Autodesk Inventor part; units mm, degrees
ref_plane "YZ Plane" through (0, 0, 0) normal (1, 0, 0) x (0, 1, 0)
ref_plane "XZ Plane" through (0, 0, 0) normal (0, 1, 0) x (-1, 0, 0)
ref_plane "XY Plane" through (0, 0, 0) normal (0, 0, 1) x (1, 0, 0)
sketch "Sketch1" plane through (0, 0, 0) normal (0, 1, 0) x (-1, 0, 0)
  circle A0 centre (0, 0) radius 76.2
  circle A1 centre (0, 0) radius 82.55
  line L0 (0, 0) -> (101.6, 0)
  arc A2 (82.55, 0) -> (101.6, 0) centre (92.075, 26.1697) ccw
  line L1 (101.6, 0) -> (92.4836, -3.3181) construction
  arc A3 (93.6625, -13.7482) -> (101.6, 0) centre (85.725, 0) ccw
  line L2 (93.6625, -13.7482) -> (79.6013, -21.8664)
  arc A4 (92.075, -10.9985) -> (98.3891, -0.9543) centre (85.725, 0) ccw
  line L3 (92.075, -10.9985) -> (80.6536, -17.5927)
  arc A5 (82.4826, -3.3343) -> (101.2144, -3.4778) centre (92.075, 26.1697) ccw
  arc A6 (-41.275, 71.4904) -> (-50.8, 87.9882) centre (-68.7011, 66.6544) ccw
  line L4 (-50.8, 87.9882) -> (-43.3683, 81.7522) construction
  arc A7 (-34.925, 87.9882) -> (-50.8, 87.9882) centre (-42.8625, 74.24) ccw
  line L5 (-34.925, 87.9882) -> (-20.8638, 79.8699)
  arc A8 (-36.5125, 85.2386) -> (-48.3681, 85.6846) centre (-42.8625, 74.24) ccw
  line L6 (-36.5125, 85.2386) -> (-25.0911, 78.6444)
  arc A9 (-38.3537, 73.0992) -> (-47.5953, 89.3931) centre (-68.7011, 66.6544) ccw
  arc A10 (-41.275, -71.4904) -> (-50.8, -87.9882) centre (-23.3739, -92.8242) ccw
  line L7 (-50.8, -87.9882) -> (-49.1154, -78.4341) construction
  arc A11 (-58.7375, -74.24) -> (-50.8, -87.9882) centre (-42.8625, -74.24) ccw
  line L8 (-58.7375, -74.24) -> (-58.7375, -58.0035)
  arc A12 (-55.5625, -74.24) -> (-50.021, -84.7303) centre (-42.8625, -74.24) ccw
  line L9 (-55.5625, -74.24) -> (-55.5625, -61.0517)
  arc A13 (-44.1289, -69.7649) -> (-53.619, -85.9153) centre (-23.3739, -92.8242) ccw
  point P0 (-20.8638, 79.8699)
  point P1 (-41.275, 71.4904)
  point P2 (-58.7375, -58.0035)
  point P3 (-41.275, -71.4904)
  point P4 (-44.1289, -69.7649)
  point P5 (-52.5943, -82.3998)
  point P6 (-55.5625, -61.0517)
  point P7 (-38.3537, 73.0992)
  point P8 (-45.0631, 86.7479)
  point P9 (-25.0911, 78.6444)
  point P10 (97.6575, -4.3481)
  dimension "d0" = 152.4
  dimension "d1" = 6.35
  dimension "d2" = 101.6
  dimension "d3" = 20
  dimension "d4" = 15.875
  dimension "d5" = 30
  dimension "d10" = 3.175
  dimension "d11" = 3.175
  dimension "d14" = 360
extrude "Extrusion1" add sketch "Sketch1" along normal blind 12.7 contours A1 | L0 A2 | A2 A4 A5 A1 | A1 L6 A8 A9 A7 L5 | A3 A5 A4 A2 | L3 A4 A5 A3 L2 A1 | A1 A6 A8 A9 | A9 A8 A6 A7 | A10 A12 A13 A1 | A1 L9 A12 A13 A11 L8 | A10 A11 A13 A12
fillet "Fillet1" radius 3.175 15 edges at (41.275, 6.35, 71.4904) (38.3537, 6.35, 73.0992) (25.0911, 6.35, 78.6444) (45.0631, 6.35, 86.7479) (52.5943, 6.35, -82.3998) (55.5625, 6.35, -61.0517) (44.1289, 6.35, -69.7649) (41.275, 6.35, -71.4904) (-79.6013, 6.35, -21.8664) (-80.6536, 6.35, -17.5927) (-82.4826, 6.35, -3.3343) (-97.6575, 6.35, -4.3481) (-82.55, 6.35, 0) (58.7375, 6.35, -58.0035) (20.8638, 6.35, 79.8699)
equation "\"d10\" = d11"
properties part number "Ring" material "Stainless Steel"
For this review, take the finished solid that the model builds, in its own axes (mm). A direction names the side the tool comes from. Round coordinates to 2 decimals unless told otherwise and drop trailing zeros. Write each loop counter-clockwise with the first axis right and the second up, starting at its lowest first coordinate (ties: lowest second). Pieces come first, ordered by that corner, then holes. Notation, with made-up numbers: (-21, -22) - (-6, -22) arc R20 ccw to (-6, 13) - close; hole circle Ø7 at (-28.5, 82.5). An arc over 180 degrees is marked (long way). Write item = value, one per line. Start each with the question number.
1. Wall thickness on L1, parallel to Z at x = 0, y = 4.5; L2, parallel to Z at x = 32.5, y = 1.5; L3, parallel to X at y = 9.5, z = -25: over which ranges is each line inside the solid? List them lowest first.
2. Consider section A-A on x = 0. State the section outline as (y, z) points.
3. For faces 5 (the face through (-36.4, 0, 67.4)), 6 (the face through (48.13, 6.26, -80.07)), 7 (the face through (33.786, 6.261, 83.665)), list the 3-axis set-ups (+Z, -Z, +X, -X, +Y, -Y) from which the entire face can be reached by the end or side of a thin tool; tool diameter is ignored.
4. Consider section B-B on z = -33.5. State the section outline as (x, y) points.
5. For pin 1 Ø6.5 at (y, z) = (7.5, -63.5) entering from +X; pin 2 Ø2 at (x, y) = (12, 9) entering from +Z; pin 3 Ø5 at (y, z) = (8, -72) entering from -X, all flat-tipped, find the tip position at first contact; note any pin that passes through.
6. Draft analysis for pull direction Z (two halves, no side actions). For faces 1 (the face through (-88.53, 6.26, -4.65)), 2 (the face through (29.406, 6.439, 79.035)), 3 (the face through (-87.281, 6.261, -17.433)), 4 (the face through (58.738, 6, -67)), state which applies: released by +Z, released by -Z, zero draft, split by the parting line, or undercut.
7. Consider section C-C on y = 7.25. Give the number of separate pieces and of enclosed holes in the cut face, plus the area to 3 significant figures.
Evaluation:
q1.L1 = -82.55 to -76.2, 76.2 to 82.55
q1.L2 = -75.88 to -68.92, 68.92 to 75.88, 82.92 to 86.59
q1.L3 = -78.67 to -71.98, 71.98 to 78.67
q2.outline = (0, -82.55) - (12.7, -82.55) - (12.7, -76.2) - (0, -76.2) - close; (0, 76.2) - (12.7, 76.2) - (12.7, 82.55) - (0, 82.55) - close
q3.face_5 = +Z, -Z, +X, -X, -Y
q3.face_6 = -Z, +Y, -Y
q3.face_7 = +Y, -Y
q4.outline = (-75.45, 0) - (-68.44, 0) - (-68.44, 12.7) - (-75.45, 12.7) - close; (68.44, 0) - (75.45, 0) - (75.45, 12.7) - (68.44, 12.7) - close
q5.pin_1 = 58.74
q5.pin_2 = 81.81
q5.pin_3 = -44.54
q6.face_1 = undercut
q6.face_2 = undercut
q6.face_3 = released by -Z
q6.face_4 = zero draft
q7.separate_pieces = 1
q7.enclosed_holes = 4
q7.area = 3,700 mm2
